Autodesk Inventor part; units mm, degrees
ref_plane "YZ Plane" through (0, 0, 0) normal (1, 0, 0) x (0, 1, 0)
ref_plane "XZ Plane" through (0, 0, 0) normal (0, 1, 0) x (-1, 0, 0)
ref_plane "XY Plane" through (0, 0, 0) normal (0, 0, 1) x (1, 0, 0)
sketch "Sketch1" plane through (0, 0, 0) normal (0, 1, 0) x (-1, 0, 0)
  line L0 (0, 0) -> (38.1, 0)
  line L1 (38.1, 0) -> (38.1, -93.98)
  line L2 (38.1, -93.98) -> (0, -93.98)
  line L3 (0, -93.98) -> (0, 0)
  dimension "d0" = 93.98
  dimension "d1" = 38.1
extrude "Extrusion1" add sketch "Sketch1" along normal blind 3.175
sketch "Sketch2" plane through (0, 3.175, 0) normal (0, 1, 0) x (1, 0, 0)
  circle A0 centre (-7.112, 8.255) radius 1.7145
  line L0 (-38.1, 0) -> (0, 0)
  line L1 (0, 0) -> (0, 93.98)
  circle A1 centre (-30.988, 8.255) radius 1.7145
  circle A2 centre (-7.112, 85.725) radius 1.7145
  circle A3 centre (-30.988, 85.725) radius 1.7145
  circle A4 centre (-14.4272, 6.604) radius 1.7145
  circle A5 centre (-22.4028, 6.604) radius 1.7145
  circle A6 centre (-14.4272, 87.376) radius 1.7145
  circle A7 centre (-22.4028, 87.376) radius 1.7145
  circle A8 centre (-5.461, 17.3482) radius 1.7145
  circle A9 centre (-5.461, 27.0256) radius 1.7145
  circle A10 centre (-5.461, 36.703) radius 1.7145
  circle A11 centre (-5.461, 46.3804) radius 1.7145
  circle A12 centre (-5.461, 56.0578) radius 1.7145
  circle A13 centre (-5.461, 65.7352) radius 1.7145
  circle A14 centre (-5.461, 75.4126) radius 1.7145
  circle A15 centre (-32.639, 17.3482) radius 1.7145
  circle A16 centre (-32.639, 27.0256) radius 1.7145
  circle A17 centre (-32.639, 36.703) radius 1.7145
  circle A18 centre (-32.639, 46.3804) radius 1.7145
  circle A19 centre (-32.639, 56.0578) radius 1.7145
  circle A20 centre (-32.639, 65.7352) radius 1.7145
  circle A21 centre (-32.639, 75.4126) radius 1.7145
  dimension "d4" = 3.429
  dimension "d5" = 8.255
  dimension "d6" = 7.112
  dimension "d9" = 23.876
  dimension "d12" = 77.47
  dimension "d15" = 14.4272
  dimension "d16" = 6.604
  dimension "d19" = 7.9756
  dimension "d22" = 80.772
  dimension "d25" = 5.461
  dimension "d26" = 17.3482
  dimension "d29" = 9.6774
  dimension "d32" = 27.178
extrude "Extrusion2" cut sketch "Sketch2" against normal through all
sketch "Sketch3" plane through (0, 0, 0) normal (0, -1, 0) x (1, 0, 0)
  line L0 (-2.54, -3.556) -> (-35.56, -3.556)
  line L1 (-35.56, -3.556) -> (-35.56, -90.424)
  line L2 (-35.56, -90.424) -> (-2.54, -90.424)
  line L3 (-2.54, -90.424) -> (-2.54, -3.556)
  circle A0 centre (-14.4272, -87.376) radius 1.7145 construction
  circle A1 centre (-5.461, -75.4126) radius 1.7145 construction
  line L4 (-38.1, -93.98) -> (0, -93.98) construction
  circle A2 centre (-14.4272, -6.604) radius 1.7145 construction
  point P0 (0, 0)
  point P1 (-19.05, -90.424)
  point P2 (-19.05, -93.98)
  dimension "d37" = 33.02
  dimension "d38" = 3.048
  dimension "d39" = 3.048
extrude "Extrusion3" add sketch "Sketch3" along normal blind 1.016
fillet "Fillet1" radius 1.27 4 edges at (-35.56, -0.508, -3.556) (-35.56, -0.508, -90.424) (-2.54, -0.508, -90.424) (-2.54, -0.508, -3.556)
sketch "Sketch4" plane through (0, 0, 0) normal (0, -1, 0) x (1, 0, 0)
  arc A0 (-2.54, -4.826) -> (-3.81, -3.556) centre (-3.81, -4.826) ccw
  line L0 (-3.81, -3.556) -> (-34.29, -3.556)
  arc A1 (-34.29, -3.556) -> (-35.56, -4.826) centre (-34.29, -4.826) ccw
  line L1 (-35.56, -4.826) -> (-35.56, -89.154)
  arc A2 (-35.56, -89.154) -> (-34.29, -90.424) centre (-34.29, -89.154) ccw
  line L2 (-34.29, -90.424) -> (-3.81, -90.424)
  arc A3 (-3.81, -90.424) -> (-2.54, -89.154) centre (-3.81, -89.154) ccw
  line L3 (-2.54, -89.154) -> (-2.54, -4.826)
  arc A4 (-0.508, -4.826) -> (-3.81, -1.524) centre (-3.81, -4.826) ccw
  line L4 (-3.81, -1.524) -> (-34.29, -1.524)
  arc A5 (-34.29, -1.524) -> (-37.592, -4.826) centre (-34.29, -4.826) ccw
  line L5 (-37.592, -4.826) -> (-37.592, -89.154)
  arc A6 (-37.592, -89.154) -> (-34.29, -92.456) centre (-34.29, -89.154) ccw
  line L6 (-34.29, -92.456) -> (-3.81, -92.456)
  arc A7 (-3.81, -92.456) -> (-0.508, -89.154) centre (-3.81, -89.154) ccw
  line L7 (-0.508, -89.154) -> (-0.508, -4.826)
  point P0 (0, 0)
  dimension "d43" = 2.032
extrude "Extrusion4" cut sketch "Sketch4" against normal blind 1.27
fillet "Fillet2" radius 1.27 4 edges at (-38.1, 1.5875, -93.98) (0, 1.5875, -93.98) (-38.1, 1.5875, 0) (0, 1.5875, 0)
sketch "Sketch5" plane through (0, 3.175, 0) normal (0, 1, 0) x (1, 0, 0)
  arc A0 (-1.27, 0) -> (0, 1.27) centre (-1.27, 1.27) ccw
  line L0 (0, 1.27) -> (0, 92.71)
  arc A1 (0, 92.71) -> (-1.27, 93.98) centre (-1.27, 92.71) ccw
  line L1 (-1.27, 93.98) -> (-36.83, 93.98)
  arc A2 (-36.83, 93.98) -> (-38.1, 92.71) centre (-36.83, 92.71) ccw
  line L2 (-38.1, 92.71) -> (-38.1, 1.27)
  arc A3 (-38.1, 1.27) -> (-36.83, 0) centre (-36.83, 1.27) ccw
  line L3 (-36.83, 0) -> (-1.27, 0)
  circle A4 centre (-32.639, 65.7352) radius 1.7145
  circle A5 centre (-32.639, 46.3804) radius 1.7145
  circle A6 centre (-32.639, 27.0256) radius 1.7145
  circle A7 centre (-5.461, 75.4126) radius 1.7145
  circle A8 centre (-5.461, 56.0578) radius 1.7145
  circle A9 centre (-5.461, 36.703) radius 1.7145
  circle A10 centre (-5.461, 17.3482) radius 1.7145
  circle A11 centre (-14.4272, 87.376) radius 1.7145
  circle A12 centre (-14.4272, 6.604) radius 1.7145
  circle A13 centre (-7.112, 85.725) radius 1.7145
  circle A14 centre (-7.112, 8.255) radius 1.7145
  circle A15 centre (-30.988, 8.255) radius 1.7145
  circle A16 centre (-30.988, 85.725) radius 1.7145
  circle A17 centre (-22.4028, 6.604) radius 1.7145
  circle A18 centre (-22.4028, 87.376) radius 1.7145
  circle A19 centre (-5.461, 27.0256) radius 1.7145
  circle A20 centre (-5.461, 46.3804) radius 1.7145
  circle A21 centre (-5.461, 65.7352) radius 1.7145
  circle A22 centre (-32.639, 17.3482) radius 1.7145
  circle A23 centre (-32.639, 36.703) radius 1.7145
  circle A24 centre (-32.639, 56.0578) radius 1.7145
  circle A25 centre (-32.639, 75.4126) radius 1.7145
  point P0 (0, 0)
extrude "Extrusion5" cut sketch "Sketch5" against normal through all contours A4 | A5 | A6 | A7 | A8 | A9 | A10 | A11 | A12 | A13 | A14 | A15 | A16 | A17 | A18 | A19 | A20 | A21 | A22 | A23 | A24 | A25
equation "\"d39\" = d38"
properties part number "TopCover" material "ABS Plastic"
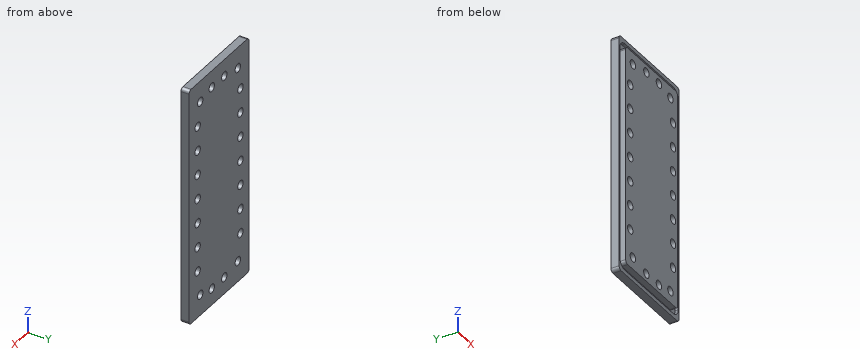
Here's how the part is built. I have some questions about the finished solid (model axes, mm). Coordinates: 2 decimals unless noted, no trailing zeros. Write each loop counter-clockwise with the first axis right and the second up, starting at its lowest first coordinate (ties: lowest second). Pieces come first, ordered by that corner, then holes. Notation, with made-up numbers: M -10,64 L -3,64 A22 cw -3,90 Z; hole C 28,19 d10. An arc over 180 degrees is marked long. Answer as CSV lines item,"result". Start each with the question number.
Q1. Suppose I cut it at B-B, the plane z = -41.5. List the corners of the cut face in (x, y) for me (3 decimals), then the cut area to 3 significant figures.
Q2. Suppose I cut it at A-A, the plane x = -27. List the corners of the cut face in (y, z) for me (3 decimals), then the cut area to 3 significant figures.
Q3. I need wall thicknesses on probe 1 along X at (y, z) = (0.25, -39); probe 2 along X at (y, z) = (2.5, -46.5); probe 3 along Z at (x, y) = (-9.5, 0.6). Which ranges of each line are inside material? Lowest first, please. Write a range as [from, to].
Q4. Suppose I cut it at C-C, the plane y = 2.2. State how many separate pieces and enclosed holes the cut face has, then the cut area to 3 significant figures.
Q5. Will this pin go through, and if not, where does the flat tip stop? pin 1 Ø2 at (x, y) = (-30.5, 2) entering from +Z.
Entries:
1,outline,"M -38.1,0 L -37.592,0 L -37.592,1.27 L -35.56,1.27 L -35.56,-1.016 L -2.54,-1.016 L -2.54,1.27 L -0.508,1.27 L -0.508,0 L 0,0 L 0,3.175 L -38.1,3.175 Z"
1,area,"149 mm²"
2,outline,"M -1.016,-90.424 L 1.27,-90.424 L 1.27,-92.456 L 0,-92.456 L 0,-93.98 L 3.175,-93.98 L 3.175,0 L 0,0 L 0,-1.524 L 1.27,-1.524 L 1.27,-3.556 L -1.016,-3.556 Z"
2,area,"381 mm²"
3,probe 1,"x = [-38.1, -37.59], [-35.56, -2.54], [-0.51, 0]"
3,probe 2,"x = [-38.1, -34.35], [-30.93, -7.17], [-3.75, 0]"
3,probe 3,"z = [-93.98, -92.46], [-90.42, -3.56], [-1.52, 0]"
4,separate pieces,"1"
4,enclosed holes,"22"
4,area,"3,380 mm²"
5,pin 1,"stops at z = 0"
